Here's how the part is built. I have some questions about the finished solid (model axes, mm). A direction names the side the tool comes from. Give positions to 0.01 mm unless a question says otherwise; leave off trailing zeros. Write each loop counter-clockwise with the first axis right and the second up, starting at its lowest first coordinate (ties: lowest second). Pieces come first, ordered by that corner, then holes. Notation, with made-up numbers: (-6.5, 58) -> (25.5, 58) arc R18 ccw to (25.5, 64) -> close; hole circle Ø4 at (57.25, -18). An arc over 180 degrees is marked (long way). Use CSV: the item, a comma, the result in double quotes. Start each with the question number.
(1) I need wall thicknesses on L1, parallel to X at y = 0, z = 16; L2, parallel to Y at x = -80, z = 2; L3, parallel to Y at x = -24, z = 21.5. Which ranges of each line are inside material? Lowest first, please. Write a range as [from, to].
(2) Suppose I cut it at D-D on x = -76. List the corners of the cut face in (y, z) for me.
(3) For pin 1 Ø1 at (x, z) = (1, 15) entering from -Y; pin 2 Ø1 at (x, y) = (61, 28.5) entering from +Z; pin 3 Ø1.5 at (x, z) = (60.5, 15) entering from -Y; pin 4 Ø4 at (x, y) = (80, 0) entering from -Z, each with a flat end and sliding along its axis, tell me the tip position at first contact or that it passes through.
(4) Suppose I cut it at A-A on x = 4.5. List the corners of the cut face in (y, z) for me.
(5) Which directions (+Z, -Z, +X, -X, +Y, -Y) give clear straight access to the entire face, cutting with the end or side of a thin tool? Please do faces 4 (the flat face through (-72.95, -18.18, 2.46)), 5 (the flat face through (61.95, -20.29, 5)).
(6) If we mould it in two halves opening along X, with no side actions, what happens to faces 1 (the cylindrical face through (62.17, 2.74, 17.26)), 2 (the flat face through (72.95, 18.18, 2.46)), 3 (the cylindrical face through (1.2, 69.57, 2.46))? For each: pulls with the +X half, pulls with the -X half, needs draft (parallel to the pull), parting line crosses it, or undercut.
(7) Suppose I cut it at B-B on y = 60. List the corners of the cut face in (x, z) for me.
(8) Suppose I cut it at C-C on z = 3. List the corners of the cut face in (x, y) for me, plus the area to 3 significant figures.
from build123d import *

# Parameters (mm, degrees)
F1_DEPTH = 5
F0_R     = 1.6686337588
F2_DEPTH = 5
F3_DEPTH = 35


with BuildPart() as f1:
    # F0 (on Top) → F1 (new body)
    with BuildSketch(Plane.XY):
        with BuildLine():
            ThreePointArc((58.9908692784, -27.2961048829), (63.4799436952, -13.9748613035), (65, 0))
            ThreePointArc((65, 0), (63.4799436952, 13.9748613035), (58.9908692784, 27.2961048829))
            ThreePointArc((58.9908692784, 27.2961048829), (35.0053794624, 54.7688178501), (0, 65))
            ThreePointArc((0, 65), (-35.0053794624, 54.7688178501), (-58.9908692784, 27.2961048829))
            ThreePointArc((-58.9908692784, 27.2961048829), (-63.4799436952, 13.9748613035), (-65, 0))
            ThreePointArc((-65, 0), (-63.4799436952, -13.9748613035), (-58.9908692784, -27.2961048829))
            ThreePointArc((-58.9908692784, -27.2961048829), (0, -65), (58.9908692784, -27.2961048829))
        make_face()
        with BuildLine():
            ThreePointArc((-62.231150434, 0), (-44.0040684729, 44.0040684729), (0, 62.231150434))
            ThreePointArc((0, 62.231150434), (44.0040684729, 44.0040684729), (62.231150434, 0))
            ThreePointArc((62.231150434, 0), (0, -62.231150434), (-62.231150434, 0))
        make_face(mode=Mode.SUBTRACT)
        with BuildLine():
            ThreePointArc((58.9908692784, 27.2961048829), (63.4799436952, 13.9748613035), (65, 0))
            Line((65, 0), (66.4206601738, 0))
            ThreePointArc((66.4206601738, 0), (67.1091179562, 4.268914411), (69.1046831796, 8.1049701726))
            ThreePointArc((69.1046831796, 8.1049701726), (67.8057771791, 15.6052670592), (65.6953330705, 22.9187912336))
            Line((65.6953330705, 22.9187912336), (58.9908692784, 27.2961048829))
        make_face()
        with BuildLine():
            Line((66.4206601738, 0), (65, 0))
            ThreePointArc((65, 0), (63.4799436952, -13.9748613035), (58.9908692784, -27.2961048829))
            Line((58.9908692784, -27.2961048829), (65.6953330705, -22.9187912336))
            ThreePointArc((65.6953330705, -22.9187912336), (67.8057771791, -15.6052670592), (69.1046831796, -8.1049701726))
            ThreePointArc((69.1046831796, -8.1049701726), (67.1091179562, -4.268914411), (66.4206601738, 0))
        make_face()
        with BuildLine():
            ThreePointArc((0, 65), (35.0053794624, 54.7688178501), (58.9908692784, 27.2961048829))
            Line((58.9908692784, 27.2961048829), (65.6953330705, 22.9187912336))
            ThreePointArc((65.6953330705, 22.9187912336), (0, 69.5783571152), (-65.6953330705, 22.9187912336))
            Line((-65.6953330705, 22.9187912336), (-58.9908692784, 27.2961048829))
            ThreePointArc((-58.9908692784, 27.2961048829), (-35.0053794624, 54.7688178501), (0, 65))
        make_face()
        with BuildLine():
            ThreePointArc((69.1046831796, 8.1049701726), (67.1091179562, 4.268914411), (66.4206601738, 0))
            ThreePointArc((66.4206601738, 0), (67.1091179562, -4.268914411), (69.1046831796, -8.1049701726))
            ThreePointArc((69.1046831796, -8.1049701726), (69.4598376886, -4.0593998478), (69.5783571152, 0))
            ThreePointArc((69.5783571152, 0), (69.4598376886, 4.0593998478), (69.1046831796, 8.1049701726))
        make_face()
        with BuildLine():
            Line((65.6953330705, -22.9187912336), (58.9908692784, -27.2961048829))
            ThreePointArc((58.9908692784, -27.2961048829), (0, -65), (-58.9908692784, -27.2961048829))
            Line((-58.9908692784, -27.2961048829), (-65.6953330705, -22.9187912336))
            ThreePointArc((-65.6953330705, -22.9187912336), (0, -69.5783571152), (65.6953330705, -22.9187912336))
        make_face()
        with BuildLine():
            Line((-65.6953330705, -22.9187912336), (-58.9908692784, -27.2961048829))
            ThreePointArc((-58.9908692784, -27.2961048829), (-63.4799436952, -13.9748613035), (-65, 0))
            Line((-65, 0), (-66.4206601738, 0))
            ThreePointArc((-66.4206601738, 0), (-67.1091179562, -4.268914411), (-69.1046831796, -8.1049701726))
            ThreePointArc((-69.1046831796, -8.1049701726), (-67.8057771791, -15.6052670592), (-65.6953330705, -22.9187912336))
        make_face()
        with BuildLine():
            ThreePointArc((-65, 0), (-63.4799436952, 13.9748613035), (-58.9908692784, 27.2961048829))
            Line((-58.9908692784, 27.2961048829), (-65.6953330705, 22.9187912336))
            ThreePointArc((-65.6953330705, 22.9187912336), (-67.8057771791, 15.6052670592), (-69.1046831796, 8.1049701726))
            ThreePointArc((-69.1046831796, 8.1049701726), (-67.1091179562, 4.268914411), (-66.4206601738, 0))
            Line((-66.4206601738, 0), (-65, 0))
        make_face()
        with BuildLine():
            ThreePointArc((-66.4206601738, 0), (-67.1091179562, 4.268914411), (-69.1046831796, 8.1049701726))
            ThreePointArc((-69.1046831796, 8.1049701726), (-69.5783571152, 0), (-69.1046831796, -8.1049701726))
            ThreePointArc((-69.1046831796, -8.1049701726), (-67.1091179562, -4.268914411), (-66.4206601738, 0))
        make_face()
    extrude(amount=F1_DEPTH)

    # F0 (on Top) → F2 (join)
    with BuildSketch(Plane.XY):
        with BuildLine():
            ThreePointArc((-69.1046831796, 8.1049701726), (-67.8057771791, 15.6052670592), (-65.6953330705, 22.9187912336))
            Line((-65.6953330705, 22.9187912336), (-80, 13.5793398262))
            ThreePointArc((-80, 13.5793398262), (-73.9033482197, 12.133808437), (-69.1046831796, 8.1049701726))
        make_face()
        with BuildLine():
            ThreePointArc((-69.1046831796, 8.1049701726), (-73.9033482197, 12.133808437), (-80, 13.5793398262))
            ThreePointArc((-80, 13.5793398262), (-89.6020432751, 9.6020432751), (-93.5793398262, 0))
            ThreePointArc((-93.5793398262, 0), (-89.6020432751, -9.6020432751), (-80, -13.5793398262))
            ThreePointArc((-80, -13.5793398262), (-73.9033482197, -12.133808437), (-69.1046831796, -8.1049701726))
            ThreePointArc((-69.1046831796, -8.1049701726), (-69.5783571152, 0), (-69.1046831796, 8.1049701726))
        make_face()
        with Locations((-80, 0)):
            Circle(F0_R, mode=Mode.SUBTRACT)
        with BuildLine():
            Line((-80, -13.5793398262), (-65.6953330705, -22.9187912336))
            ThreePointArc((-65.6953330705, -22.9187912336), (-67.8057771791, -15.6052670592), (-69.1046831796, -8.1049701726))
            ThreePointArc((-69.1046831796, -8.1049701726), (-73.9033482197, -12.133808437), (-80, -13.5793398262))
        make_face()
        with BuildLine():
            ThreePointArc((80, -13.5793398262), (73.9033482197, -12.133808437), (69.1046831796, -8.1049701726))
            ThreePointArc((69.1046831796, -8.1049701726), (67.8057771791, -15.6052670592), (65.6953330705, -22.9187912336))
            Line((65.6953330705, -22.9187912336), (80, -13.5793398262))
        make_face()
        with BuildLine():
            ThreePointArc((80, 13.5793398262), (73.9033482197, 12.133808437), (69.1046831796, 8.1049701726))
            ThreePointArc((69.1046831796, 8.1049701726), (69.4598376886, 4.0593998478), (69.5783571152, 0))
            ThreePointArc((69.5783571152, 0), (69.4598376886, -4.0593998478), (69.1046831796, -8.1049701726))
            ThreePointArc((69.1046831796, -8.1049701726), (73.9033482197, -12.133808437), (80, -13.5793398262))
            ThreePointArc((80, -13.5793398262), (89.6020432751, -9.6020432751), (93.5793398262, 0))
            ThreePointArc((93.5793398262, 0), (89.6020432751, 9.6020432751), (80, 13.5793398262))
        make_face()
        with Locations((80, 0)):
            Circle(F0_R, mode=Mode.SUBTRACT)
        with BuildLine():
            Line((80, 13.5793398262), (65.6953330705, 22.9187912336))
            ThreePointArc((65.6953330705, 22.9187912336), (67.8057771791, 15.6052670592), (69.1046831796, 8.1049701726))
            ThreePointArc((69.1046831796, 8.1049701726), (73.9033482197, 12.133808437), (80, 13.5793398262))
        make_face()
    extrude(amount=F2_DEPTH)

    # F0 (on Top) → F3 (join)
    with BuildSketch(Plane.XY):
        with BuildLine():
            ThreePointArc((58.9908692784, -27.2961048829), (63.4799436952, -13.9748613035), (65, 0))
            ThreePointArc((65, 0), (63.4799436952, 13.9748613035), (58.9908692784, 27.2961048829))
            ThreePointArc((58.9908692784, 27.2961048829), (35.0053794624, 54.7688178501), (0, 65))
            ThreePointArc((0, 65), (-35.0053794624, 54.7688178501), (-58.9908692784, 27.2961048829))
            ThreePointArc((-58.9908692784, 27.2961048829), (-63.4799436952, 13.9748613035), (-65, 0))
            ThreePointArc((-65, 0), (-63.4799436952, -13.9748613035), (-58.9908692784, -27.2961048829))
            ThreePointArc((-58.9908692784, -27.2961048829), (0, -65), (58.9908692784, -27.2961048829))
        make_face()
        with BuildLine():
            ThreePointArc((-62.231150434, 0), (-44.0040684729, 44.0040684729), (0, 62.231150434))
            ThreePointArc((0, 62.231150434), (44.0040684729, 44.0040684729), (62.231150434, 0))
            ThreePointArc((62.231150434, 0), (0, -62.231150434), (-62.231150434, 0))
        make_face(mode=Mode.SUBTRACT)
    extrude(amount=F3_DEPTH)


solid = f1.part
Geometry says:
1,L1,"[-65, -62.23], [62.23, 65]"
1,L2,"[-13.58, -1.67], [1.67, 13.58]"
1,L3,"[-60.41, -57.42], [57.42, 60.41]"
2,outline,"(-16.19, 0) -> (16.19, 0) -> (16.19, 5) -> (-16.19, 5) -> close"
3,pin 1,"y = -65"
3,pin 2,"z = 5"
3,pin 3,"y = -25.59"
3,pin 4,"z = 0"
4,outline,"(-69.43, 0) -> (-62.07, 0) -> (-62.07, 35) -> (-64.84, 35) -> (-64.84, 5) -> (-69.43, 5) -> close; (62.07, 0) -> (69.43, 0) -> (69.43, 5) -> (64.84, 5) -> (64.84, 35) -> (62.07, 35) -> close"
5,face 4,"+Z, -Z, -X, -Y"
5,face 5,"+Z"
6,face 1,"undercut"
6,face 2,"pulls with the +X half"
6,face 3,"parting line crosses it"
7,outline,"(-35.23, 0) -> (-16.51, 0) -> (-16.51, 35) -> (-25, 35) -> (-25, 5) -> (-35.23, 5) -> close; (16.51, 0) -> (35.23, 0) -> (35.23, 5) -> (25, 5) -> (25, 35) -> (16.51, 35) -> close"
8,outline,"(-80, -13.58) -> (-65.7, -22.92) arc R69.58 ccw to (65.7, -22.92) -> (80, -13.58) arc R13.58 ccw to (80, 13.58) -> (65.7, 22.92) arc R69.58 ccw to (-65.7, 22.92) -> (-80, 13.58) arc R13.58 ccw to start; hole circle Ø3.34 at (-80, 0); hole circle Ø124.46 at (0, 0); hole circle Ø3.34 at (80, 0)"
8,area,"4,410 mm²"
